Could you check a few things on this model? Use its own coordinates, in mm. A direction names the side the tool comes from. Round coordinates to 2 decimals unless told otherwise and drop trailing zeros. Loops run counter-clockwise (first coordinate to the right, second up) from the corner with the lowest first, then second, coordinate; pieces in that order, holes last. Notation, with made-up numbers: (-39, 89.25) - (-27, 89.25) arc R13 ccw to (-27, 99.25) - close; hole circle Ø9 at (23, -40). An arc over 180 degrees is marked (long way). Answer as CSV lines item,"result". Start each with the question number.
1) Suppose I cut it at B-B, the plane x = -4. Write out the boundary of the cut face in (y, z), then the cut area to 3 significant figures.
2) Please list where these lines run through material, in increasing order: line 1 along X through (y, z) = (14, -4.25); line 2 along X through (y, z) = (10.75, -9); line 3 along Y through (x, z) = (7.2, -7.1).
3) I'm going to push flat-ended pins straight in: pin 1 Ø10 at (x, y) = (3.5, 20) entering from -Z; pin 2 Ø2 at (x, z) = (1.5, -11) entering from +Y; pin 3 Ø1.2 at (x, y) = (0, -2.5) entering from +Z; pin 4 Ø0.8 at (x, y) = (5.5, 14.5) entering from +Z. Where does each tip first touch, or does it pass through?
4) Suppose I cut it at C-C, the plane y = 7.25. Write out the boundary of the cut face in (x, z), then the cut area to 4 significant figures.
5) Suppose I cut it at D-D, the plane z = -13. Write out the boundary of the cut face in (x, y).
6) Suppose I cut it at A-A, the plane z = -5.5. Write out the boundary of the cut face in (x, y).
7) Which directions (+Z, -Z, +X, -X, +Y, -Y) give clear straight access to the entire face, cutting with the end or side of a thin tool? Please do faces 1 (the face through (-5.5, -1, -24)), 2 (the face through (3.9, -2.3, -19.5)), 3 (the face through (-8, 18, -5.1)).
8) We'd pull the mould along Y, two halves only. Please class faces 4 (the face through (6.4, 15, -10)), 5 (the face through (6.98, 18.39, -7.22)), 6 (the face through (0, 0, -19)): pulls with the +Y half, pulls with the -Y half, needs draft (parallel to the pull), parting line crosses it, or undercut.
```python
from build123d import *

# Parameters (mm, degrees)
EXTRUDE_1_DEPTH     = 25
SKETCH_2_W          = 19
SKETCH_2_H          = 28
EXTRUDE_2_DEPTH     = 3
SKETCH_3_W          = 1
SKETCH_3_H          = 6
CUT_EXTRUDE_1_DEPTH = 15
CUT_EXTRUDE_START   = -19
SKETCH_4_R          = 0.9
CUT_EXTRUDE_2_DEPTH = 19
FILLET_1_R          = 3
EXTRUDE_3_DEPTH     = 1.5
EXTRUDE_4_DEPTH     = 5
CHAMFER_1_SIZE      = 0.5
SHELL_START         = -8
SHELL_1_DEPTH       = 16
SHELL_1_2_DEPTH     = 0.05
SHELL_START_2       = 7.95
SHELL_1_3_DEPTH     = 0.05
CUT_EXTRUDE_3_DEPTH = 1.5
SKETCH_8_W          = 12.8
SKETCH_8_H          = 20
CUT_EXTRUDE_4_DEPTH = 1.5


# Read off the part's stored shape, not the designer's step: 抽壳1
with BuildPart() as part:
    # 草图1 → 凸台-拉伸1 (new body)
    with BuildSketch(Plane(origin=(0, 0, 0), x_dir=(1, 0, 0), z_dir=(0, 1, 0))):
        Polygon((-9.5, 11.1), (-9.5, 0), (9.5, 0), (9.5, 11.1), (4.95, 11.1), (4.95, 8.1), (6.45, 8.1), (6.45, 2), (-6.45, 2), (-6.45, 8.1), (-4.95, 8.1), (-4.95, 11.1), align=None)
    extrude(amount=EXTRUDE_1_DEPTH)

    # 草图2 → 凸台-拉伸2 (add)
    with BuildSketch(Plane.XZ):
        with Locations((0, -14)):
            Rectangle(SKETCH_2_W, SKETCH_2_H)
        with BuildLine():
            Line((-2.5, -22.5), (-2.5, -24.5))
            ThreePointArc((-2.5, -24.5), (-4, -26), (-5.5, -24.5))
            Line((-5.5, -24.5), (-5.5, -22.5))
            ThreePointArc((-5.5, -22.5), (-4, -21), (-2.5, -22.5))
        make_face(mode=Mode.SUBTRACT)
        with BuildLine():
            Line((2.5, -24.5), (2.5, -22.5))
            ThreePointArc((2.5, -22.5), (4, -21), (5.5, -22.5))
            Line((5.5, -22.5), (5.5, -24.5))
            ThreePointArc((5.5, -24.5), (4, -26), (2.5, -24.5))
        make_face(mode=Mode.SUBTRACT)
    extrude(amount=EXTRUDE_2_DEPTH)

    # 草图3 → 切除-拉伸1 (cut)
    with BuildSketch(Plane(origin=(0, 25, 0), x_dir=(1, 0, 0), z_dir=(0, 1, 0))):
        with Locations((-8, 8.1)):
            Rectangle(SKETCH_3_W, SKETCH_3_H)
        with Locations((8, 8.1)):
            Rectangle(SKETCH_3_W, SKETCH_3_H)
    extrude(amount=-CUT_EXTRUDE_1_DEPTH, mode=Mode.SUBTRACT)

    # 草图4 → 切除-拉伸2 (cut)
    with BuildSketch(Plane.ZY.offset(9.5).offset(CUT_EXTRUDE_START)):
        with Locations((-7.1, 17.5)):
            Circle(SKETCH_4_R)
    extrude(amount=CUT_EXTRUDE_2_DEPTH, mode=Mode.SUBTRACT)

    # 圆角1
    fillet_1_edges = [part.edges().sort_by_distance(p)[0] for p in [
        (9.5, -1.5, -28),
        (-9.5, -1.5, -28),
    ]]
    fillet(fillet_1_edges, radius=FILLET_1_R)

    # 草图5 → 凸台-拉伸3 (add)
    with BuildSketch(Plane.ZY.offset(9.5)):
        Polygon((-11.1, 0), (-11.1, 6), (-21.1, 0), align=None)
    extrude_3 = extrude(amount=-EXTRUDE_3_DEPTH)

    # 镜向1: 凸台-拉伸3 across plane
    add(extrude_3.mirror(Plane(origin=(0, 0, 0), x_dir=(0, 0, 1), z_dir=(1, 0, 0))))

    # 草图6 → 凸台-拉伸4 (add)
    with BuildSketch(Plane(origin=(0, 0, 0), x_dir=(1, 0, 0), z_dir=(0, 1, 0))):
        Polygon((-6.45, 2), (6.45, 2), (6.45, 8.1), (4.95, 8.1), (4.95, 11.1), (-4.95, 11.1), (-4.95, 8.1), (-6.45, 8.1), align=None)
    extrude(amount=EXTRUDE_4_DEPTH)

    # 倒角1
    chamfer_1_edges = [part.edges().sort_by_distance(p)[0] for p in [
        (4.95, 25, -9.6),
        (5.7, 25, -8.1),
        (6.45, 25, -5.05),
        (0, 25, -2),
        (-6.45, 25, -5.05),
        (-5.7, 25, -8.1),
        (-4.95, 25, -9.6),
    ]]
    chamfer(chamfer_1_edges, length=CHAMFER_1_SIZE)

    # 抽壳1 outline → 抽壳1 (cut)
    with BuildSketch(Plane.YZ.offset(SHELL_START)):
        Polygon((3.5, -0.5), (23.5, -0.5), (23.5, 0), (-1.5, 0), (-1.5, -9.6), (3.5, -9.6), align=None)
    extrude(amount=SHELL_1_DEPTH, mode=Mode.SUBTRACT)

    # Shell 1 2 outline → Shell 1 2 (cut)
    with BuildSketch(Plane.YZ.offset(SHELL_START)):
        Polygon((8.5, -3.6), (23.5, -3.6), (23.5, -0.5), (3.5, -0.5), (3.5, -9.6), (8.5, -9.6), align=None)
    extrude(amount=SHELL_1_2_DEPTH, mode=Mode.SUBTRACT)

    # Shell 1 3 outline → Shell 1 3 (cut)
    with BuildSketch(Plane.YZ.offset(SHELL_START_2)):
        Polygon((8.5, -3.6), (23.5, -3.6), (23.5, -0.5), (3.5, -0.5), (3.5, -9.6), (8.5, -9.6), align=None)
    extrude(amount=SHELL_1_3_DEPTH, mode=Mode.SUBTRACT)

    # 草图7 → 切除-拉伸3 (cut)
    with BuildSketch(Plane.XZ.offset(3)):
        with BuildLine():
            Line((8, -11.1), (-8, -11.1))
            Line((-8, -11.1), (-8, -25))
            ThreePointArc((-8, -25), (-7.560660172, -26.060660172), (-6.5, -26.5))
            Line((-6.5, -26.5), (-6.236067977, -26.5))
            ThreePointArc((-6.236067977, -26.5), (-6.802517077, -25.570466269), (-7, -24.5))
            Line((-7, -24.5), (-7, -22.5))
            ThreePointArc((-7, -22.5), (-4, -19.5), (-1, -22.5))
            Line((-1, -22.5), (-1, -24.5))
            ThreePointArc((-1, -24.5), (-1.197482923, -25.570466269), (-1.763932023, -26.5))
            Line((-1.763932023, -26.5), (1.763932023, -26.5))
            ThreePointArc((1.763932023, -26.5), (1.197482923, -25.570466269), (1, -24.5))
            Line((1, -24.5), (1, -22.5))
            ThreePointArc((1, -22.5), (4, -19.5), (7, -22.5))
            Line((7, -22.5), (7, -24.5))
            ThreePointArc((7, -24.5), (6.802517077, -25.570466269), (6.236067977, -26.5))
            Line((6.236067977, -26.5), (6.5, -26.5))
            ThreePointArc((6.5, -26.5), (7.560660172, -26.060660172), (8, -25))
            Line((8, -25), (8, -11.1))
        make_face()
    extrude(amount=-CUT_EXTRUDE_3_DEPTH, mode=Mode.SUBTRACT)

    # 草图8 → 切除-拉伸4 (cut)
    with BuildSketch(Plane(origin=(0, 0, -11.1), x_dir=(-1, 0, 0), z_dir=(0, 0, -1))):
        with Locations((0, 15)):
            Rectangle(SKETCH_8_W, SKETCH_8_H)
    extrude(amount=-CUT_EXTRUDE_4_DEPTH, mode=Mode.SUBTRACT)


solid = part.part
```
Filled sheet:
1,outline,"(-3, -28) - (0, -28) - (0, -26) - (-3, -26) - close; (-3, -21) - (0, -21) - (0, -11.1) - (5, -11.1) - (5, -2) - (24.5, -2) - (25, -1.5) - (25, 0) - (23.5, 0) - (23.5, -0.5) - (3.5, -0.5) - (3.5, -9.6) - (-1.5, -9.6) - (-1.5, 0) - (-3, 0) - (-3, -11.1) - (-1.5, -11.1) - (-1.5, -19.5) - (-3, -19.5) - close"
1,area,"93.8 mm²"
2,line 1,"-9.5 to -6.45, 6.45 to 9.5"
2,line 2,"-9.5 to -8.5, -7.5 to -4.95, 4.95 to 7.5, 8.5 to 9.5"
2,line 3,"-3 to -1.5, 3.5 to 16.6, 18.4 to 25"
3,pin 1,"z = -11.1"
3,pin 2,"y = 5"
3,pin 3,"z = 0"
3,pin 4,"z = -0.5"
4,outline,"(-9.5, -11.1) - (-6.4, -11.1) - (-6.4, -9.6) - (-4.95, -9.6) - (-4.95, -8.1) - (-6.45, -8.1) - (-6.45, -2) - (6.45, -2) - (6.45, -8.1) - (4.95, -8.1) - (4.95, -9.6) - (6.4, -9.6) - (6.4, -11.1) - (9.5, -11.1) - (9.5, 0) - (8, 0) - (8, -9.6) - (7.95, -9.6) - (7.95, -0.5) - (-7.95, -0.5) - (-7.95, -9.6) - (-8, -9.6) - (-8, 0) - (-9.5, 0) - close"
4,area,"89.25 mm²"
5,outline,"(-9.5, -3) - (-8, -3) - (-8, -1.5) - (8, -1.5) - (8, -3) - (9.5, -3) - (9.5, 4.86) - (8, 4.86) - (8, 0) - (-8, 0) - (-8, 4.86) - (-9.5, 4.86) - close"
6,outline,"(-9.5, -3) - (9.5, -3) - (9.5, 25) - (8.5, 25) - (8.5, 10) - (7.5, 10) - (7.5, 25) - (6.95, 25) - (6.45, 24.5) - (6.45, 5) - (-6.45, 5) - (-6.45, 24.5) - (-6.95, 25) - (-7.5, 25) - (-7.5, 10) - (-8.5, 10) - (-8.5, 25) - (-9.5, 25) - close; hole (-8, -1.5) - (8, -1.5) - (8, 8.5) - (7.95, 8.5) - (7.95, 3.5) - (-7.95, 3.5) - (-7.95, 8.5) - (-8, 8.5) - close"
7,face 1,"+Y, -Y"
7,face 2,"-Y"
7,face 3,"-Z, +Y"
8,face 4,"needs draft"
8,face 5,"undercut"
8,face 6,"pulls with the +Y half"
